Model file for the job. Use its own axes, mm. Face numbers are marked on the shaded views. A direction names the side the tool comes from. Round coordinates to 2 decimals unless told otherwise and drop trailing zeros. Write each loop counter-clockwise with the first axis right and the second up, starting at its lowest first coordinate (ties: lowest second). Pieces come first, ordered by that corner, then holes.
```python
from build123d import *

# Parameters (mm, degrees)
EXTRUDE_1_DEPTH          = 4
CUT_EXTRUDE_1_DEPTH      = 38.905694823
CUT_EXTRUDE_1_DEPTH_BACK = 38.905694823
SKETCH_2_R               = 1
SKETCH_3_W               = 14
SKETCH_3_H               = 20.72
CUT_EXTRUDE_3_DEPTH      = 3
SKETCH_5_W               = 5
SKETCH_5_H               = 20.72
CUT_EXTRUDE_4_DEPTH      = 4
SKETCH_13_W              = 24.72
SKETCH_13_H              = 4
EXTRUDE_5_DEPTH          = 27
SKETCH_15_R              = 10
EXTRUDE_6_DEPTH          = 4
SKETCH_14_R              = 1.5
CUT_EXTRUDE_7_DEPTH      = 4
FILLET_1_R               = 10
FILLET_2_R               = 10
SKETCH_6_R               = 11
CUT_EXTRUDE_9_DEPTH      = 4
SKETCH_17_W              = 24.72
SKETCH_17_H              = 4
CUT_EXTRUDE_10_DEPTH     = 16
FILLET_3_R               = 2
FILLET_4_R               = 2
FILLET_5_R               = 2
FILLET_6_R               = 2
SKETCH_18_R              = 3
CUT_EXTRUDE_11_DEPTH     = 13
SKETCH_20_R              = 3
CUT_EXTRUDE_12_DEPTH     = 3


with BuildPart() as part:
    # 草图1 → 凸台-拉伸1 (new body)
    with BuildSketch(Plane(origin=(0, 0, 0), x_dir=(1, 0, 0), z_dir=(0, 1, 0))):
        with BuildLine():
            Line((6.61, -12.36), (9.61, -12.36))
            Line((9.61, -12.36), (9.61, -9.36))
            Line((9.61, -9.36), (9.61, 9.36))
            Line((9.61, 9.36), (9.61, 12.36))
            Line((9.61, 12.36), (6.61, 12.36))
            Line((6.61, 12.36), (-32.61, 12.36))
            ThreePointArc((-32.61, 12.36), (-34.731320344, 11.481320344), (-35.61, 9.36))
            Line((-35.61, 9.36), (-35.61, -9.36))
            ThreePointArc((-35.61, -9.36), (-34.731320344, -11.481320344), (-32.61, -12.36))
            Line((-32.61, -12.36), (6.61, -12.36))
        make_face()
    extrude(amount=EXTRUDE_1_DEPTH)

    # 草图2 → 切除-拉伸1 (cut, two sides: drawn at the far end of the back side and taken through both)
    with BuildSketch(Plane(origin=(0, 0, 0), x_dir=(1, 0, 0), z_dir=(0, 1, 0)).offset(-CUT_EXTRUDE_1_DEPTH_BACK)):
        with Locations(Location((7.25, -10.25, 0), (0, 0, 270))):
            Circle(SKETCH_2_R)
        with Locations(Location((7.25, 10.25, 0), (0, 0, 270))):
            Circle(SKETCH_2_R)
        with Locations(Location((-17.2, -10.25, 0), (0, 0, 270))):
            Circle(SKETCH_2_R)
        with Locations(Location((-17.2, 10.25, 0), (0, 0, 270))):
            Circle(SKETCH_2_R)
    extrude(amount=CUT_EXTRUDE_1_DEPTH + CUT_EXTRUDE_1_DEPTH_BACK, mode=Mode.SUBTRACT)

    # 草图3 → 切除-拉伸3 (cut)
    with BuildSketch(Plane(origin=(0, 4, 0), x_dir=(1, 0, 0), z_dir=(0, 1, 0))):
        with Locations((-1.39, 0)):
            Rectangle(SKETCH_3_W, SKETCH_3_H)
    extrude(amount=-CUT_EXTRUDE_3_DEPTH, mode=Mode.SUBTRACT)

    # 草图5 → 切除-拉伸4 (cut)
    with BuildSketch(Plane(origin=(0, 4, 0), x_dir=(1, 0, 0), z_dir=(0, 1, 0))):
        with Locations((-10.89, 0)):
            Rectangle(SKETCH_5_W, SKETCH_5_H)
    extrude(amount=-CUT_EXTRUDE_4_DEPTH, mode=Mode.SUBTRACT)

    # 草图13 → 凸台-拉伸5 (add)
    with BuildSketch(Plane(origin=(9.61, 0, 0), x_dir=(0, 0, -1), z_dir=(1, 0, 0))):
        with Locations((0, 2)):
            Rectangle(SKETCH_13_W, SKETCH_13_H)
    extrude(amount=EXTRUDE_5_DEPTH)

    # 草图15 → 凸台-拉伸6 (add)
    with BuildSketch(Plane(origin=(0, 4, 0), x_dir=(1, 0, 0), z_dir=(0, 1, 0))):
        with Locations(Location((24.25, 0, 0), (0, 0, 270))):
            Circle(SKETCH_15_R)
    extrude(amount=EXTRUDE_6_DEPTH)

    # 草图14 → 切除-拉伸7 (cut, symmetric)
    with BuildSketch(Plane(origin=(0, 4, 0), x_dir=(1, 0, 0), z_dir=(0, 1, 0))):
        with Locations(Location((24.25, -7, 0), (0, 0, 270))):
            Circle(SKETCH_14_R)
        with Locations(Location((31.25, 0, 0), (0, 0, 270))):
            Circle(SKETCH_14_R)
        with Locations(Location((24.25, 7, 0), (0, 0, 270))):
            Circle(SKETCH_14_R)
        with Locations(Location((17.25, 0, 0), (0, 0, 270))):
            Circle(SKETCH_14_R)
    extrude(amount=CUT_EXTRUDE_7_DEPTH, both=True, mode=Mode.SUBTRACT)

    # 圆角1
    fillet_1_edges = [part.edges().sort_by_distance(p)[0] for p in [
        (36.61, 2, -12.36),
    ]]
    fillet(fillet_1_edges, radius=FILLET_1_R)

    # 圆角2
    fillet_2_edges = [part.edges().sort_by_distance(p)[0] for p in [
        (36.61, 2, 12.36),
    ]]
    fillet(fillet_2_edges, radius=FILLET_2_R)

    # 草图6 → 切除-拉伸9 (cut)
    with BuildSketch(Plane(origin=(0, 4, 0), x_dir=(1, 0, 0), z_dir=(0, 1, 0))):
        with Locations((-25.5, 0)):
            Circle(SKETCH_6_R)
    extrude(amount=-CUT_EXTRUDE_9_DEPTH, mode=Mode.SUBTRACT)

    # 草图17 → 切除-拉伸10 (cut)
    with BuildSketch(Plane.ZY.offset(35.61)):
        with Locations((0, 2)):
            Rectangle(SKETCH_17_W, SKETCH_17_H)
    extrude(amount=-CUT_EXTRUDE_10_DEPTH, mode=Mode.SUBTRACT)

    # 圆角3
    fillet_3_edges = [part.edges().sort_by_distance(p)[0] for p in [
        (-19.61, 2, 12.36),
    ]]
    fillet(fillet_3_edges, radius=FILLET_3_R)

    # 圆角4
    fillet_4_edges = [part.edges().sort_by_distance(p)[0] for p in [
        (-19.61, 2, -12.36),
    ]]
    fillet(fillet_4_edges, radius=FILLET_4_R)

    # 圆角5
    fillet_5_edges = [part.edges().sort_by_distance(p)[0] for p in [
        (-19.61, 2, -9.290204519),
    ]]
    fillet(fillet_5_edges, radius=FILLET_5_R)

    # 圆角6
    fillet_6_edges = [part.edges().sort_by_distance(p)[0] for p in [
        (-19.61, 2, 9.290204519),
    ]]
    fillet(fillet_6_edges, radius=FILLET_6_R)

    # 草图18 → 切除-拉伸11 (cut)
    with BuildSketch(Plane(origin=(0, 8, 0), x_dir=(1, 0, 0), z_dir=(0, 1, 0))):
        with Locations(Location((24.25, 0, 0), (0, 0, 270))):
            Circle(SKETCH_18_R)
    extrude(amount=-CUT_EXTRUDE_11_DEPTH, mode=Mode.SUBTRACT)

    # 草图20 → 切除-拉伸12 (cut)
    with BuildSketch(Plane.XZ):
        with Locations(Location((24.25, 7, 0), (0, 0, 270))):
            Circle(SKETCH_20_R)
        with Locations(Location((17.25, 0, 0), (0, 0, 270))):
            Circle(SKETCH_20_R)
        with Locations(Location((24.25, -7, 0), (0, 0, 270))):
            Circle(SKETCH_20_R)
        with Locations(Location((31.25, 0, 0), (0, 0, 270))):
            Circle(SKETCH_20_R)
    extrude(amount=-CUT_EXTRUDE_12_DEPTH, mode=Mode.SUBTRACT)


solid = part.part
```
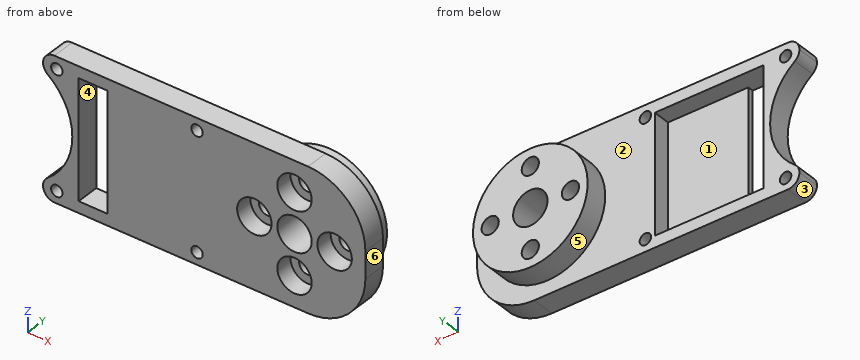
1) Pull direction Z, two halves, no side cores. Call the marked faces 1, 2 and 3: released by +Z, released by -Z, zero draft, split by the parting line, or undercut.
2) Cut at D-D on y = 2.5. Give the number of separate pieces and of enclosed holes in the cut face, and give its area (3 significant figures).
3) Cut at B-B on z = -4.5. List the corners of the cut face in (x, y).
4) Wall check: probe 1 along Z at (x, y) = (7.25, 1.7); probe 2 along X at (y, z) = (3.7, 0); probe 3 along X at (y, z) = (4.75, 0). Give the ranges that are in metal, low to high.
5) Flat gauge pins, fed straight in: pin 1 Ø5 at (x, z) = (10, 9.5) entering from +Y; pin 2 Ø2 at (y, z) = (4, 4) entering from -X; pin 3 Ø1.6 at (x, z) = (7.25, 10.25) entering from -Y; pin 4 Ø1.8 at (x, z) = (18.5, 1.5) entering from -Y. Where does each tip first touch, or does it go through?
6) Cut at A-A on x = 7.25. List the corners of the cut face in (y, z), and give its area (3 significant figures).
7) Cut at C-C on x = 18. List the corners of the cut face in (y, z).
8) Which spindle directions (+Z, -Z, +X, -X, +Y, -Y) get a long thin tool onto all of the face, cutting with end or side? Do the marked faces 4, 5 and 6. Say none if no direction does.
Result sheet:
1. face 1: undercut
1. face 2: zero draft
1. face 3: released by -Z
2. separate pieces: 1
2. enclosed holes: 10
2. area: 730 mm2
3. outline: (-15.46, 0) - (-13.39, 0) - (-13.39, 4) - (-15.46, 4) - close; (-8.39, 0) - (22.59, 0) - (22.59, 3) - (25.91, 3) - (25.91, 0) - (36.38, 0) - (36.38, 4) - (33.18, 4) - (33.18, 8) - (15.32, 8) - (15.32, 4) - (5.61, 4) - (5.61, 1) - (-8.39, 1) - close
4. probe 1: z = -12.36 to -11.25, -9.25 to 9.25, 11.25 to 12.36
4. probe 2: x = -14.5 to -13.39, 5.61 to 15.75, 18.75 to 21.25, 27.25 to 29.75, 32.75 to 36.61
4. probe 3: x = 14.25 to 15.75, 18.75 to 21.25, 27.25 to 29.75, 32.75 to 34.25
5. pin 1: stops at y = 4
5. pin 2: stops at x = -15.7
5. pin 3: passes through
5. pin 4: stops at y = 3
6. outline: (0, -12.36) - (4, -12.36) - (4, -11.25) - (0, -11.25) - close; (0, -9.25) - (4, -9.25) - (4, 9.25) - (0, 9.25) - close; (0, 11.25) - (4, 11.25) - (4, 12.36) - (0, 12.36) - close
6. area: 82.9 mm2
7. outline: (0, -12.36) - (4, -12.36) - (4, -7.81) - (8, -7.81) - (8, -1.3) - (3, -1.3) - (3, -2.9) - (0, -2.9) - close; (0, 2.9) - (3, 2.9) - (3, 1.3) - (8, 1.3) - (8, 7.81) - (4, 7.81) - (4, 12.36) - (0, 12.36) - close
8. face 4: +Y, -Y
8. face 5: +Y
8. face 6: +Z, -Z, +X, +Y, -Y
